Autodesk Inventor part; units mm, degrees
ref_plane "YZ Plane" through (0, 0, 0) normal (1, 0, 0) x (0, 1, 0)
ref_plane "XZ Plane" through (0, 0, 0) normal (0, 1, 0) x (-1, 0, 0)
ref_plane "XY Plane" through (0, 0, 0) normal (0, 0, 1) x (1, 0, 0)
sketch "Sketch1" plane through (0, 0, 0) normal (0, 1, 0) x (-1, 0, 0)
  line L0 (6, 6) -> (-6, 6)
  line L1 (-6, 6) -> (-6, -6)
  line L2 (-6, -6) -> (6, -6)
  line L3 (6, -6) -> (6, 6)
  line L4 (6, 6) -> (-6, -6) construction
  line L5 (-6, 6) -> (6, -6) construction
  point P0 (0, 0)
  dimension "d0" = 12
  dimension "d1" = 12
sketch "Sketch2" plane through (0, 0, 0) normal (0, 1, 0) x (-1, 0, 0)
  line L0 (5, -5) -> (-5, -5)
  line L1 (-5, -5) -> (-5, 15)
  line L2 (-5, 15) -> (5, 15)
  line L3 (5, 15) -> (5, -5)
  point P0 (0, 0)
  dimension "d2" = 10
  dimension "d3" = 20
extrude "Extrusion1" add sketch "Sketch1" along normal blind 22
extrude "Extrusion2" cut sketch "Sketch2" along normal blind 21
sketch "Sketch3" plane through (6, 0, 6) normal (1, 0, 0) x (0, 0, -1)
  line L0 (0, 0) -> (0, 22)
  line L1 (10, 18) -> (0, 18)
  line L2 (0, 18) -> (0, 12)
  line L3 (0, 12) -> (10, 12)
  line L4 (10, 12) -> (10, 18)
  point P0 (6, 0)
  dimension "d8" = 6
extrude "Extrusion3" cut sketch "Sketch3" against normal blind 1
sketch "Sketch4" plane through (0, 21, 0) normal (0, -1, 0) x (1, 0, 0)
  line L0 (-5, -5) -> (-5, 6)
  line L1 (-5, -5) -> (-0.5, -5)
  line L2 (-0.5, -5) -> (-0.5, -1.5)
  line L3 (-0.5, -1.5) -> (-5, -1.5)
  line L4 (-5, -1.5) -> (-5, -5)
  point P0 (0, 0)
  dimension "d11" = 4.5
  dimension "d12" = 3.5
extrude "Extrusion4" add sketch "Sketch4" along normal blind 9
properties part number "housing_v10"
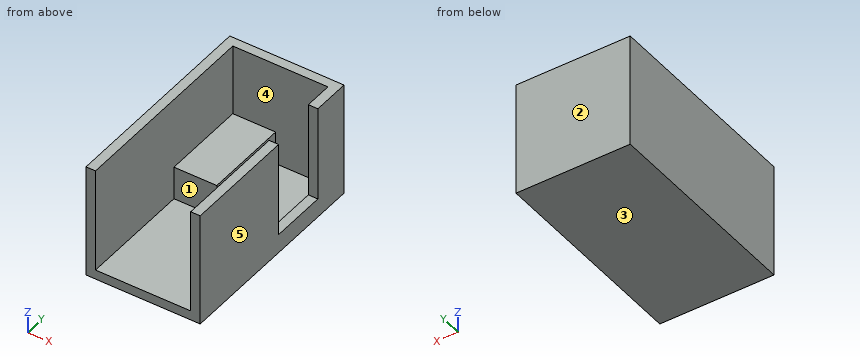
The listing builds one solid part. Answer for the finished solid, in the listing's coordinates (mm). Face numbers are marked on the shaded views. A direction names the side the tool comes from. Round coordinates to 2 decimals unless told otherwise and drop trailing zeros. Loops run counter-clockwise (first coordinate to the right, second up) from the corner with the lowest first, then second, coordinate; pieces in that order, holes last. Notation, with made-up numbers: (-20.5, -3) - (-15.5, -3) arc R33 cw to (-15.5, 34) - close; hole circle Ø11 at (44, 67). An arc over 180 degrees is marked (long way). Return JSON: item names as keys, results as strings. Group by question number.
1. The part is cut by section D-D on y = 11.25. Determine the outline of the cut face in (x, z), then the cut area to 3 significant figures.
2. The mould has two halves that part along X. Classify the marked faces 3, 4 and 5: pulls with the +X half, pulls with the -X half, needs draft (parallel to the pull), parting line crosses it, or undercut.
3. The part is cut by section B-B on y = 16.5. Determine the outline of the cut face in (x, z).
4. The part is cut by section A-A on z = -0.25. Determine the outline of the cut face in (x, y), then the cut area to 3 significant figures.
5. Each of these flat-tipped pins is pushed along its axis until it touches: P1, Ø1.5, axis at x = -1, y = 17, coming from the +Z side; P2, Ø4, axis at x = -2, z = 4, coming from the -Y side; P3, Ø1.1, axis at x = 5.5, y = 15, coming from the +Z side. Where does it stop, or does it pass through?
6. Consider probe 1 along X at (y, z) = (7.5, 2); probe 2 along X at (y, z) = (19.75, -4.75); probe 3 along Y at (x, z) = (5.25, -2.75). Determine where each line is inside the solid, lowest interval first.
7. The part is cut by section C-C on x = -2.75. Determine the outline of the cut face in (y, z).
8. Which of the six approach directions +Z, -Z, +X, -X, +Y, -Y give full straight-line access (tool end or side, diameter ignored) to the marked faces 1 and 2?
Resolved:
{
 "1": {"outline": "(-6, -6) - (6, -6) - (6, 6) - (5, 6) - (5, -5) - (-5, -5) - (-5, 6) - (-6, 6) - close", "area": "34.0 mm²"},
 "2": {"face 3": "needs draft", "face 4": "undercut", "face 5": "pulls with the +X half"},
 "3": {"outline": "(-6, -6) - (6, -6) - (6, -4) - (5, -4) - (5, -5) - (-0.5, -5) - (-0.5, -1.5) - (-5, -1.5) - (-5, 6) - (-6, 6) - close"},
 "4": {"outline": "(-6, 0) - (-5, 0) - (-5, 21) - (5, 21) - (5, 18) - (6, 18) - (6, 22) - (-6, 22) - close; (5, 0) - (6, 0) - (6, 12) - (5, 12) - close", "area": "48.0 mm²"},
 "5": {"P1": "stops at z = -1.5", "P2": "stops at y = 21", "P3": "stops at z = -4"},
 "6": {"probe 1": "x = -6 to -5, 5 to 6", "probe 2": "x = -6 to -0.5, 5 to 6", "probe 3": "y = 0 to 12, 18 to 22"},
 "7": {"outline": "(0, -6) - (22, -6) - (22, 6) - (21, 6) - (21, -1.5) - (12, -1.5) - (12, -5) - (0, -5) - close"},
 "8": {"face 1": "+Z, -Y", "face 2": "+Z, -Z, +X, -X, +Y"}
}
